from build123d import *

# Parameters (mm, degrees)
SKETCH_1_W          = 28
SKETCH_1_H          = 47
EXTRUDE_1_DEPTH     = 17
EXTRUDE_2_DEPTH     = 2.5
SKETCH_3_W          = 32
SKETCH_3_H          = 51
EXTRUDE_3_DEPTH     = 2
SKETCH_5_W          = 1.5
SKETCH_5_H          = 4
CUT_EXTRUDE_3_DEPTH = 10
SKETCH_6_W          = 24
SKETCH_6_H          = 15
EXTRUDE_4_DEPTH     = 1
SKETCH_7_W          = 20
SKETCH_7_H          = 10
EXTRUDE_5_DEPTH     = 1
EXTRUDE_6_DEPTH     = 10
SKETCH_9_R          = 2.25
CUT_EXTRUDE_4_DEPTH = 20.5
FILLET_1_R          = 3


with BuildPart() as part:
    # Эскиз1 → Бобышка-Вытянуть1 (new body)
    with BuildSketch(Plane.XY):
        with Locations((14, 23.5)):
            Rectangle(SKETCH_1_W, SKETCH_1_H)
    extrude(amount=EXTRUDE_1_DEPTH)

    # Эскиз2 → Бобышка-Вытянуть2 (add)
    with BuildSketch(Plane.XY.offset(17)):
        Polygon((-4, 53), (32, 53), (43.5, 23.5), (32, -6), (-4, -6), (-15.5, 23.5), align=None)
    extrude(amount=EXTRUDE_2_DEPTH)

    # Эскиз3 → Бобышка-Вытянуть3 (add)
    with BuildSketch(Plane.XY.offset(19.5)):
        with Locations((14, 23.5)):
            Rectangle(SKETCH_3_W, SKETCH_3_H)
    extrude(amount=EXTRUDE_3_DEPTH)

    # Эскиз5 → Вырез-Вытянуть3 (cut)
    with BuildSketch(Plane.XY.offset(21.5)):
        Polygon((2, 18), (26, 18), (26, 8), (20, 2), (8, 2), (2, 8), align=None)
        with Locations((8, 13)):
            Rectangle(SKETCH_5_W, SKETCH_5_H, mode=Mode.SUBTRACT)
        with Locations((14, 9)):
            Rectangle(SKETCH_5_W, SKETCH_5_H, mode=Mode.SUBTRACT)
        with Locations((20, 13)):
            Rectangle(SKETCH_5_W, SKETCH_5_H, mode=Mode.SUBTRACT)
    extrude(amount=-CUT_EXTRUDE_3_DEPTH, mode=Mode.SUBTRACT)

    # Эскиз6 → Бобышка-Вытянуть4 (add)
    with BuildSketch(Plane.XY.offset(21.5)):
        with Locations((14, 36.5)):
            Rectangle(SKETCH_6_W, SKETCH_6_H)
    extrude(amount=EXTRUDE_4_DEPTH)

    # Эскиз7 → Бобышка-Вытянуть5 (add)
    with BuildSketch(Plane.XY.offset(22.5)):
        with Locations((14, 36.5)):
            Rectangle(SKETCH_7_W, SKETCH_7_H)
    extrude(amount=EXTRUDE_5_DEPTH)

    # Эскиз8 → Бобышка-Вытянуть6 (add)
    with BuildSketch(Plane.XZ.offset(-31.5)):
        with BuildLine():
            Line((4, 23.5), (24, 23.5))
            ThreePointArc((24, 23.5), (15.801732114, 24.706928456), (8, 27.5))
            ThreePointArc((8, 27.5), (5.80973161, 25.69026839), (4, 23.5))
        make_face()
    extrude(amount=-EXTRUDE_6_DEPTH)

    # Эскиз9 → Вырез-Вытянуть4 (cut, through all)
    with BuildSketch(Plane.XY.offset(19.5)):
        with Locations((-6, 23.5)):
            Circle(SKETCH_9_R)
        with Locations((34, 23.5)):
            Circle(SKETCH_9_R)
    extrude(amount=-CUT_EXTRUDE_4_DEPTH, mode=Mode.SUBTRACT)

    # Скругление1
    fillet_1_edges = [part.edges().sort_by_distance(p)[0] for p in [
        (43.5, 23.5, 18.25),
        (32, 53, 18.25),
        (-4, 53, 18.25),
        (-15.5, 23.5, 18.25),
        (-4, -6, 18.25),
        (32, -6, 18.25),
        (0, 47, 8.5),
        (28, 47, 8.5),
        (28, 0, 8.5),
        (0, 0, 8.5),
    ]]
    fillet(fillet_1_edges, radius=FILLET_1_R)


solid = part.part
Verification items for the finished model (mm, model axes). A direction names the side the tool comes from. Coordinates: 2 decimals unless noted, no trailing zeros. Order: outer loops, then holes, each group sorted by start corner. A loop starts at its lowest first (then second) coordinate and runs counter-clockwise, first axis right, second up.
1. Sectioned sample at C-C, the plane z = 3. Record the cut outline in (x, y), and give its area (3 significant figures).
Results found:
outline: (0, 3) arc R3 ccw to (3, 0) - (25, 0) arc R3 ccw to (28, 3) - (28, 44) arc R3 ccw to (25, 47) - (3, 47) arc R3 ccw to (0, 44) - close
area: 1,310 mm2
2. Go/stop test with flat-tipped pins: pin 1 Ø8 at (x, y) = (35.5, 41.5) entering from -Z; pin 2 Ø0.8 at (x, z) = (12, 22) entering from -Y; pin 3 Ø8 at (x, z) = (-1, 11.5) entering from +Y. Record where each tip stops, or that it passes through.
Results found:
pin 1: stops at z = 17
pin 2: stops at y = 29
pin 3: stops at y = 47
3. Set-up check for faces 4 (the face through (12, 31.5, 24)), 5 (the face through (0.86, 46.1, 8.62)), 6 (the face through (14, 11, 17)), 7 (the face through (-2, 23, 20)), 8 (the face through (-5, 30, 17)): record each of +Z, -Z, +X, -X, +Y, -Y from which the full face is reachable in a straight line by a thin tool's end or side.
Results found:
face 4: +Z, +X, -X, -Y
face 5: -Z, -X, +Y
face 6: +Z
face 7: +Z, -X, +Y, -Y
face 8: -Z
4. Sectioned sample at B-B, the plane z = 14.75. Record the cut outline in (x, y), and give its area (3 significant figures).
Results found:
outline: (0, 3) arc R3 ccw to (3, 0) - (25, 0) arc R3 ccw to (28, 3) - (28, 44) arc R3 ccw to (25, 47) - (3, 47) arc R3 ccw to (0, 44) - close; (7.25, 11) - (8.75, 11) - (8.75, 15) - (7.25, 15) - close; (13.25, 7) - (14.75, 7) - (14.75, 11) - (13.25, 11) - close; (19.25, 11) - (20.75, 11) - (20.75, 15) - (19.25, 15) - close; hole (2, 8) - (8, 2) - (20, 2) - (26, 8) - (26, 18) - (2, 18) - close
area: 978 mm2
5. Scan lines: line 1 (Z direction, x = 31.5, y = 22.5); line 2 (Z direction, x = 29.5, y = 31); line 3 (X direction, y = 22, z = 8). Record each from-to range of solid material in increasing order.
Results found:
line 1: z = 17 to 19.5
line 2: z = 17 to 21.5
line 3: x = 0 to 28
6. Sectioned sample at A-A, the plane z = 18.25. Give the number of separate pieces and of enclosed holes in the cut face, and give its area (3 significant figures).
Results found:
separate pieces: 4
enclosed holes: 3
area: 2,440 mm2
7. Release check for a two-part mould opening along X. For faces 1 (the face through (14, 42, 22.5)), 2 (the face through (20, 15, 17)), 3 (the face through (-15.28, 23.52, 18.27)) record: +X half, -X half, draft (parallel to the pull), parting line (faces both ways), or undercut.
Results found:
face 1: draft
face 2: undercut
face 3: -X half
8. Sectioned sample at D-D, the plane y = 27. Record the cut outline in (x, z), and give its area (3 significant figures).
Results found:
outline: (-14.14, 17) - (0, 17) - (0, 0) - (28, 0) - (28, 17) - (42.14, 17) - (42.14, 19.5) - (30, 19.5) - (30, 21.5) - (-2, 21.5) - (-2, 19.5) - (-14.14, 19.5) - close
area: 681 mm2
